The model under review builds one solid part; all positions refer to its coordinate system, in mm. A direction names the side the tool comes from. Coordinates: 2 decimals unless noted, no trailing zeros. Loops run counter-clockwise (first coordinate to the right, second up) from the corner with the lowest first, then second, coordinate; pieces in that order, holes last. Notation, with made-up numbers: M 0.25,-36.5 L 49.25,-36.5 A18 ccw 49.25,-28.5 Z; hole C 15,38 d7. An arc over 180 degrees is marked long. Return JSON: item names as keys, results as strings.
```python
from build123d import *

# Parameters (mm, degrees)
EXTRUDE_1_DEPTH     = 22
SKETCH_4_W          = 1
SKETCH_4_H          = 22
EXTRUDE_2_DEPTH     = 1
SKETCH_2_W          = 1
SKETCH_2_H          = 22
EXTRUDE_3_DEPTH     = 1
CUT_EXTRUDE_2_DEPTH = 5


with BuildPart() as part:
    # Эскиз1 → Бобышка-Вытянуть1 (new body)
    with BuildSketch(Plane.XY):
        with BuildLine():
            Line((19.485571585, 11.25), (22.516660498, 13))
            ThreePointArc((22.516660498, 13), (26, 0), (22.516660498, -13))
            Line((22.516660498, -13), (19.485571585, -11.25))
            ThreePointArc((19.485571585, -11.25), (22.5, 0), (19.485571585, 11.25))
        make_face()
    extrude(amount=EXTRUDE_1_DEPTH)

    # Эскиз4 → Бобышка-Вытянуть2 (add)
    with BuildSketch(Plane(origin=(0, 0, 0), x_dir=(-0.866025403784438, -0.5000000000000012, 0), z_dir=(-0.5000000000000011, 0.8660254037844379, 0))):
        with Locations((-24.25, 11)):
            Rectangle(SKETCH_4_W, SKETCH_4_H)
    extrude(amount=EXTRUDE_2_DEPTH)

    # Эскиз2 → Бобышка-Вытянуть3 (add)
    with BuildSketch(Plane(origin=(0, 0, 0), x_dir=(0.866025403784438, -0.5000000000000012, 0), z_dir=(-0.5000000000000011, -0.8660254037844379, 0))):
        with Locations((24.25, 11)):
            Rectangle(SKETCH_2_W, SKETCH_2_H)
    extrude(amount=EXTRUDE_3_DEPTH)

    # Эскиз6 → Вырез-Вытянуть2 (cut)
    with BuildSketch(Plane(origin=(0, 0, 0), x_dir=(-1, 0, 0), z_dir=(0, 0, -1))):
        with BuildLine():
            Line((-21.733331092, 5.823428515), (-25.114071484, 6.729295173))
            ThreePointArc((-25.114071484, 6.729295173), (-26, 0), (-25.114071484, -6.729295173))
            Line((-25.114071484, -6.729295173), (-21.733331092, -5.823428515))
            ThreePointArc((-21.733331092, -5.823428515), (-22.5, 0), (-21.733331092, 5.823428515))
        make_face()
    extrude(amount=-CUT_EXTRUDE_2_DEPTH, mode=Mode.SUBTRACT)


solid = part.part
```
1. Machinability: for faces 5 (the face through (22, 12.7, 10.8)), 6 (the face through (22, -9, 0)), 7 (the face through (21.19, -12.8, 10.85)), 8 (the face through (24, 0, 5)), 9 (the face through (20.034, -11.567, 10.846)), which of the approach directions +Z, -Z, +X, -X, +Y, -Y give a long, thin tool a straight path to every point of the face, cutting with its end or side? Answer none if there is none.
Check values:
{"face 5": "+Z, -Z, +Y", "face 6": "-Z, +X, -X, +Y, -Y", "face 7": "+Z, -Z, -Y", "face 8": "-Z, +X", "face 9": "+Z, -Z, -X"}
2. Add section B-B on x = 24.5. Give the boundary of the cut face in (y, z), plus the area to 3 significant figures.
Check values:
{"outline": "M -8.7,0 L -6.56,0 L -6.56,5 L 6.56,5 L 6.56,0 L 8.7,0 L 8.7,22 L -8.7,22 Z", "area": "317 mm²"}
3. To check wall thickness, follow line 1 (Y direction, x = 20.5, z = 15.5); line 2 (Z direction, x = 25, y = -4); line 3 (Y direction, x = 20.75, z = 14.5). State the ranges of each line that lie inside material, in increasing order.
Check values:
{"line 1": "-12.99 to -11.99, -11.84 to -9.27, 9.27 to 11.84, 11.99 to 12.99", "line 2": "5 to 22", "line 3": "-13.13 to -8.7, 8.7 to 13.13"}
4. Add section D-D on y = -1.75. Give the boundary of the cut face in (x, z).
Check values:
{"outline": "M 22.43,5 L 25.94,5 L 25.94,22 L 22.43,22 Z"}
5. Insertion check: pin 1 Ø4 at (y, z) = (-6, 18.5) entering from +X; pin 2 Ø1.5 at (y, z) = (-8.5, 16) entering from +X; pin 3 Ø2 at (y, z) = (9, 9) entering from +X. Each pin has a flat end and moves straight along its axis. Give the tip position at first contact, or say it passes through.
Check values:
{"pin 1": "x = 25.69", "pin 2": "x = 24.82", "pin 3": "x = 24.74"}
6. The part is to be moulded in two halves that separate along X. For faces 1 (the face through (20.5, -12.99, 11.15)), 2 (the face through (23.447, -6.283, 2.465)), 3 (the face through (21.19, 12.8, 10.85)), 4 (the face through (22, -12.7, 10.8)), say which applies: released by +X, released by -X, zero draft, split by the parting line, or undercut.
Check values:
{"face 1": "released by -X", "face 2": "released by +X", "face 3": "undercut", "face 4": "undercut"}
7. Add section C-C on z = 13. Give the boundary of the cut face in (x, y) (3 decimals).
Check values:
{"outline": "M 19.486,-11.25 L 20.568,-11.875 L 20.068,-12.741 L 20.934,-13.241 L 21.434,-12.375 L 22.517,-13 A26 ccw 22.517,13 L 21.434,12.375 L 20.934,13.241 L 20.068,12.741 L 20.568,11.875 L 19.486,11.25 A22.5 cw Z"}
8. Add section A-A on z = 2.5. Give the boundary of the cut face in (x, y) (3 decimals), plus the area to 3 significant figures.
Check values:
{"outline": "M 19.486,-11.25 L 20.568,-11.875 L 20.068,-12.741 L 20.934,-13.241 L 21.434,-12.375 L 22.517,-13 A26 ccw 25.114,-6.729 L 21.733,-5.823 A22.5 cw Z; M 19.486,11.25 A22.5 cw 21.733,5.823 L 25.114,6.729 A26 ccw 22.517,13 L 21.434,12.375 L 20.934,13.241 L 20.068,12.741 L 20.568,11.875 Z", "area": "46.4 mm²"}
